Input: part model. Units: mm. Frame: model coordinates. A direction names the side the tool comes from. Coordinates: 2 decimals unless noted, no trailing zeros. Order: outer loops, then holes, each group sorted by start corner. A loop starts at its lowest first (then second) coordinate and runs counter-clockwise, first axis right, second up. Notation, with made-up numbers: (-15.75, 73) -> (32.25, 73) arc R21 ccw to (32.25, 100) -> close; hole circle Ø4 at (47, 87). An arc over 180 degrees is marked (long way). Answer as CSV lines item,"result".
Solid Edge part; units mm, degrees
sketch "Sketch1" plane through (0, 0, 0) normal (0, 0, 1) x (1, 0, 0)
  circle A0 centre (0, 0) radius 2.5
extrude "Protrusion1" add sketch "Sketch1" along normal blind 3
sketch "Sketch2" plane through (0, 0, 0) normal (1, 0, 0) x (0, 1, 0)
  circle A0 centre (0, 1.5) radius 1
extrude "ExtrudedCutout_1" add sketch "Sketch2" along normal mid plane 7.2
sketch "Sketch3" plane through (0, 0, 0) normal (0, -1, 0) x (1, 0, 0)
  circle A0 centre (0, 1.5) radius 1
extrude "ExtrudedProtrusion_3" add sketch "Sketch3" along normal mid plane 7.2
1. Cut plane C-C (z = 1.5). Return the cut outline in (x, y).
Findings:
outline,"(-3.6, -1) -> (-2.29, -1) arc R2.5 ccw to (-1, -2.29) -> (-1, -3.6) -> (1, -3.6) -> (1, -2.29) arc R2.5 ccw to (2.29, -1) -> (3.6, -1) -> (3.6, 1) -> (2.29, 1) arc R2.5 ccw to (1, 2.29) -> (1, 3.6) -> (-1, 3.6) -> (-1, 2.29) arc R2.5 ccw to (-2.29, 1) -> (-3.6, 1) -> close"
2. Cut plane D-D (z = 0.75). Return the cut outline in (x, y).
Findings:
outline,"(-3.6, -0.66) -> (-2.41, -0.66) arc R2.5 ccw to (-0.66, -2.41) -> (-0.66, -3.6) -> (0.66, -3.6) -> (0.66, -2.41) arc R2.5 ccw to (2.41, -0.66) -> (3.6, -0.66) -> (3.6, 0.66) -> (2.41, 0.66) arc R2.5 ccw to (0.66, 2.41) -> (0.66, 3.6) -> (-0.66, 3.6) -> (-0.66, 2.41) arc R2.5 ccw to (-2.41, 0.66) -> (-3.6, 0.66) -> close"
3. Ray query, line 1 along X through (y, z) = (2.5, 1.5); line 2 along X through (y, z) = (1, 2.2). Return the intervals inside material, ascending.
Findings:
line 1,"x = -1 to 1"
line 2,"x = -2.29 to 2.29"
4. Cut plane A-A (x = 0). Return the cut outline in (y, z), plus the area to 3 significant figures.
Findings:
outline,"(-3.6, 0.5) -> (-2.5, 0.5) -> (-2.5, 0) -> (2.5, 0) -> (2.5, 0.5) -> (3.6, 0.5) -> (3.6, 2.5) -> (2.5, 2.5) -> (2.5, 3) -> (-2.5, 3) -> (-2.5, 2.5) -> (-3.6, 2.5) -> close"
area,"19.4 mm2"
5. Reachability of faces 1 (the face through (1.15, 2.22, 1.48)), 2 (the face through (-2.936, 0.924, 1.117)), 3 (the face through (0.924, 2.936, 1.117)), 4 (the face through (0.924, -2.936, 1.883)), 5 (the face through (2.936, 0.924, 1.883)) from +Z, -Z, +X, -X, +Y, -Y: full face, straight path, thin tool, end or side. Return the list, or none.
Findings:
face 1,"none"
face 2,"-X"
face 3,"+Y"
face 4,"-Y"
face 5,"+X"
